Input: part model. Units: mm. Frame: model coordinates. A direction names the side the tool comes from. Give positions to 0.01 mm unless a question says otherwise; leave off trailing zeros. Loops run counter-clockwise (first coordinate to the right, second up) from the corner with the lowest first, then second, coordinate; pieces in that order, holes last. Notation, with made-up numbers: (69, 17) - (81, 17) arc R23 ccw to (81, 34) - close; hole circle Ø8 at (85.25, -7.5). An arc over 180 degrees is marked (long way). Answer as a JSON object with one key per item and string values.
from build123d import *

# Parameters (mm, degrees)
SKETCH7_R                      = 1.75
CUT_EXTRUDE1_DEPTH             = 22.664170882
CBORE_FOR_M3_SHCS1_D           = 3.2
CBORE_FOR_M3_SHCS1_CBORE_D     = 6
CBORE_FOR_M3_SHCS1_CBORE_DEPTH = 3


with BuildPart() as part:
    # Sketch2 → Revolve1 (revolve)
    with BuildSketch(Plane.XY):
        Polygon((0, 0), (0, 12.87), (1, 12.87), (1, 11.87), (10.75, 11.87), (10.75, 12.87), (11.75, 12.87), (11.75, 0), align=None)
    revolve(axis=Axis((11.75, 0, 0), (-1, 0, 0)))

    # Sketch7 → Cut-Extrude1 (cut, through all)
    with BuildSketch(Plane(origin=(11.75, 0, 0), x_dir=(0, 0, -1), z_dir=(1, 0, 0))):
        with Locations(Location((0, 0, 0), (0, 0, 90))):
            Circle(SKETCH7_R)
    extrude(amount=-CUT_EXTRUDE1_DEPTH, mode=Mode.SUBTRACT)

    # CBORE for M3 SHCS1 (through all)
    with Locations(Plane(origin=(11.75, 0, 0), x_dir=(0, 0, -1), z_dir=(1, 0, 0))):
        with Locations((0, -4), (0, 4)):
            CounterBoreHole(CBORE_FOR_M3_SHCS1_D / 2, CBORE_FOR_M3_SHCS1_CBORE_D / 2, CBORE_FOR_M3_SHCS1_CBORE_DEPTH)


solid = part.part
Item 1: Cut plane B-B (x = 3). Return loops of the section in (y, z).
Geometry check:
{"outline": "circle Ø23.74 at (0, 0); hole circle Ø3.2 at (-4, 0); hole circle Ø3.5 at (0, 0); hole circle Ø3.2 at (4, 0)"}
Item 2: Material intervals for line 1 (Y direction, x = 6.5, z = 0); line 2 (Z direction, x = 9, y = 0); line 3 (Z direction, x = 9.6, y = 4), sorted ascending. Write a range as [from, to].
Geometry check:
{"line 1": "y = [-11.87, -5.6], [-2.4, -1.75], [1.75, 2.4], [5.6, 11.87]", "line 2": "z = [-11.87, -1.75], [1.75, 11.87]", "line 3": "z = [-11.18, -3], [3, 11.18]"}
Item 3: Access query for faces 1 (the face through (11.75, 0, 3)), 2 (the face through (1, 8.5, 8.5)), 3 (the face through (8.75, 5.4, -1.3)). Directions: +Z, -Z, +X, -X, +Y, -Y. A direction counts if a zero-diameter tool reaches every point of the face in a straight line with its end or side. Return the directions, or none.
Geometry check:
{"face 1": "+Z, -Z, +X, +Y, -Y", "face 2": "none", "face 3": "+X"}
Item 4: Mould query, pull axis Z, two halves, no side actions, for faces 4 (the face through (0.507, -2.79, 12.564)), 5 (the face through (10.75, -8.5, 8.5)), 6 (the face through (5.957, 1.617, -0.67)). Classes: released by +Z, released by -Z, zero draft, split by the parting line, or undercut.
Geometry check:
{"face 4": "split by the parting line", "face 5": "zero draft", "face 6": "undercut"}
Item 5: Contact query for flat-ended pins moving along their axis: P1, Ø5, axis at x = 1.5, z = 6.5, coming from the +Y side; P2, Ø6, axis at x = 10.5, y = -10, coming from the +Z side; P3, Ø2.5, axis at y = 4, z = 0, coming from the -X side; P4, Ø6, axis at x = 10, y = -7.5, coming from the +Z side. Output: stop coordinate, or through.
Geometry check:
{"P1": "stops at y = 12.22", "P2": "stops at z = 10.79", "P3": "passes through", "P4": "stops at z = 12.02"}
Item 6: Cut plane D-D (y = 4). Return loops of the section in (x, z).
Geometry check:
{"outline": "(0, -12.23) - (1, -12.23) - (1, -11.18) - (10.75, -11.18) - (10.75, -12.23) - (11.75, -12.23) - (11.75, -3) - (8.75, -3) - (8.75, -1.6) - (0, -1.6) - close; (0, 1.6) - (8.75, 1.6) - (8.75, 3) - (11.75, 3) - (11.75, 12.23) - (10.75, 12.23) - (10.75, 11.18) - (1, 11.18) - (1, 12.23) - (0, 12.23) - close"}
Item 7: Cut plane C-C (z = 10.5). Return loops of the section in (x, y).
Geometry check:
{"outline": "(0, -7.44) - (1, -7.44) - (1, -5.54) - (10.75, -5.54) - (10.75, -7.44) - (11.75, -7.44) - (11.75, 7.44) - (10.75, 7.44) - (10.75, 5.54) - (1, 5.54) - (1, 7.44) - (0, 7.44) - close"}
Item 8: Cut plane A-A (y = 0). Return loops of the section in (x, z).
Geometry check:
{"outline": "(0, -12.87) - (1, -12.87) - (1, -11.87) - (10.75, -11.87) - (10.75, -12.87) - (11.75, -12.87) - (11.75, -1.75) - (0, -1.75) - close; (0, 1.75) - (11.75, 1.75) - (11.75, 12.87) - (10.75, 12.87) - (10.75, 11.87) - (1, 11.87) - (1, 12.87) - (0, 12.87) - close"}
